Autodesk Inventor part; units mm, degrees
ref_plane "YZ Plane" through (0, 0, 0) normal (1, 0, 0) x (0, 1, 0)
ref_plane "XZ Plane" through (0, 0, 0) normal (0, 1, 0) x (-1, 0, 0)
ref_plane "XY Plane" through (0, 0, 0) normal (0, 0, 1) x (1, 0, 0)
sketch "Skizze1" plane through (0, 0, 0) normal (0, 0, 1) x (1, 0, 0)
  line L0 (-22.5, -22.5) -> (22.5, -22.5)
  line L1 (22.5, -22.5) -> (22.5, 22.5)
  line L2 (22.5, 22.5) -> (-22.5, 22.5)
  line L3 (-22.5, 22.5) -> (-22.5, -22.5)
  line L4 (-22.5, -22.5) -> (22.5, 22.5) construction
  line L5 (22.5, -22.5) -> (-22.5, 22.5) construction
  point P0 (0, 0)
  dimension "d0" = 45
  dimension "d1" = 45
extrude "Extrusion1" add sketch "Skizze1" along normal blind 7
sketch "Skizze2" plane through (0, 0, 0) normal (0, 0, -1) x (-1, 0, 0)
  line L0 (-22.5, -22.5) -> (-22.5, 22.5)
  line L1 (-22.5, 22.5) -> (22.5, 22.5)
  line L2 (22.5, 22.5) -> (22.5, -22.5)
  line L3 (22.5, -22.5) -> (-22.5, -22.5)
  point P0 (0, 0)
  point P1 (-17.5, 17.5)
  point P2 (17.5, 17.5)
  point P3 (17.5, -17.5)
  point P4 (-17.5, -17.5)
  dimension "d4" = 5
  dimension "d5" = 5
  dimension "d6" = 5
  dimension "d7" = 5
  dimension "d8" = 5
  dimension "d9" = 5
  dimension "d12" = 5
  dimension "d13" = 5
hole "Bohrung1" at (17.5, 17.5, 0) at (-17.5, 17.5, 0) at (-17.5, -17.5, 0) at (17.5, -17.5, 0) direction (0, 0, 1) diameter 4 end through all
sketch "Skizze3" plane through (0, 0, 0) normal (0, 0, -1) x (-1, 0, 0)
  line L0 (-22.5, 22.5) -> (22.5, 22.5)
  line L1 (-22.5, 22.5) -> (-12.5, 22.5)
  line L2 (-12.5, 22.5) -> (-12.5, 12.5)
  line L3 (-12.5, 12.5) -> (-22.5, 12.5)
  line L4 (-22.5, 12.5) -> (-22.5, 22.5)
  line L5 (22.5, 22.5) -> (12.5, 22.5)
  line L6 (12.5, 22.5) -> (12.5, 12.5)
  line L7 (12.5, 12.5) -> (22.5, 12.5)
  line L8 (22.5, 12.5) -> (22.5, 22.5)
  line L9 (22.5, 22.5) -> (22.5, -22.5)
  line L10 (22.5, -22.5) -> (12.5, -22.5)
  line L11 (12.5, -22.5) -> (12.5, -12.5)
  line L12 (12.5, -12.5) -> (22.5, -12.5)
  line L13 (22.5, -12.5) -> (22.5, -22.5)
  line L14 (22.5, -22.5) -> (-22.5, -22.5)
  line L15 (-22.5, -22.5) -> (-12.5, -22.5)
  line L16 (-12.5, -22.5) -> (-12.5, -12.5)
  line L17 (-12.5, -12.5) -> (-22.5, -12.5)
  line L18 (-22.5, -12.5) -> (-22.5, -22.5)
  point P0 (0, 0)
  dimension "d21" = 10
  dimension "d22" = 10
  dimension "d23" = 10
  dimension "d24" = 10
  dimension "d25" = 10
  dimension "d26" = 10
  dimension "d27" = 10
properties part number "Platte klein"
Work out the finished part from the listing and answer in its coordinate system (mm). Round coordinates to 2 decimals unless told otherwise and drop trailing zeros. Write each loop counter-clockwise with the first axis right and the second up, starting at its lowest first coordinate (ties: lowest second). Pieces come first, ordered by that corner, then holes.
1) A cutting plane is placed at A-A (x = 17.5). Give the vertices of the cut face in (y, z).
2) Given pin 1 Ø4.5 at (x, y) = (-17.5, -17.5) entering from +Z; pin 2 Ø3.5 at (x, y) = (17.5, -17.5) entering from +Z, each flat-ended and moving along its own axis, determine where each tip first touches the part or whether it passes through.
3) Straight lines are drawn through the part: line 1 (X direction, y = -17.5, z = 2); line 2 (X direction, y = 17, z = 0.75). For each, find the intervals that lie inside material, in ascending order.
4) The mould has two halves that part along X. Classify faces 1 (the flat face through (0, 0, 0)), 2 (the flat face through (-22.5, 0, 3)), 3 (the flat face through (22.5, 0, 3)), 4 (the cylindrical face through (15.517, -17.76, 3.549)): pulls with the +X half, pulls with the -X half, needs draft (parallel to the pull), parting line crosses it, or undercut.
5) A cutting plane is placed at C-C (z = 5). Give the vertices of the cut face in (x, y).
Completed:
1. outline: (-22.5, 0) - (-19.5, 0) - (-19.5, 7) - (-22.5, 7) - close; (-15.5, 0) - (15.5, 0) - (15.5, 7) - (-15.5, 7) - close; (19.5, 0) - (22.5, 0) - (22.5, 7) - (19.5, 7) - close
2. pin 1: stops at z = 7
2. pin 2: passes through
3. line 1: x = -22.5 to -19.5, -15.5 to 15.5, 19.5 to 22.5
3. line 2: x = -22.5 to -19.44, -15.56 to 15.56, 19.44 to 22.5
4. face 1: needs draft
4. face 2: pulls with the -X half
4. face 3: pulls with the +X half
4. face 4: undercut
5. outline: (-22.5, -22.5) - (22.5, -22.5) - (22.5, 22.5) - (-22.5, 22.5) - close; hole circle Ø4 at (-17.5, -17.5); hole circle Ø4 at (-17.5, 17.5); hole circle Ø4 at (17.5, -17.5); hole circle Ø4 at (17.5, 17.5)
